from build123d import *

# Parameters (mm, degrees)
SKETCH1_W           = 165
SKETCH1_H           = 50.84
BOSS_EXTRUDE1_DEPTH = 10
SKETCH2_W           = 90
SKETCH2_H           = 10
BOSS_EXTRUDE2_DEPTH = 110
SKETCH3_R           = 4
CUT_EXTRUDE1_DEPTH  = 30
SKETCH4_W           = 90
SKETCH4_H           = 110
CUT_EXTRUDE2_DEPTH  = 0.5


with BuildPart() as part:
    # Sketch1 → Boss-Extrude1 (new body)
    with BuildSketch(Plane(origin=(0, 0, 0), x_dir=(1, 0, 0), z_dir=(0, 1, 0))):
        with Locations((82.5, 25.42)):
            Rectangle(SKETCH1_W, SKETCH1_H)
    extrude(amount=BOSS_EXTRUDE1_DEPTH)

    # Sketch2 → Boss-Extrude2 (add)
    with BuildSketch(Plane(origin=(0, 10, 0), x_dir=(1, 0, 0), z_dir=(0, 1, 0))):
        with Locations((80, 45.84)):
            Rectangle(SKETCH2_W, SKETCH2_H)
        with Locations((80, 5)):
            Rectangle(SKETCH2_W, SKETCH2_H)
    extrude(amount=BOSS_EXTRUDE2_DEPTH)

    # Sketch3 → Cut-Extrude1 (cut)
    with BuildSketch(Plane(origin=(0, 10, 0), x_dir=(1, 0, 0), z_dir=(0, 1, 0))):
        with Locations((30, 36.92)):
            Circle(SKETCH3_R)
        with Locations((155, 36.92)):
            Circle(SKETCH3_R)
    cut_extrude1 = extrude(amount=-CUT_EXTRUDE1_DEPTH, mode=Mode.SUBTRACT)

    # Mirror1: Cut-Extrude1 across plane
    add(cut_extrude1.mirror(Plane(origin=(0, 0, -25.42), x_dir=(1, 0, 0), z_dir=(0, 0, -1))), mode=Mode.SUBTRACT)

    # Sketch4 → Cut-Extrude2 (cut)
    with BuildSketch(Plane(origin=(0, 0, -10), x_dir=(-1, 0, 0), z_dir=(0, 0, -1))):
        with Locations((-80, 65)):
            Rectangle(SKETCH4_W, SKETCH4_H)
    cut_extrude2 = extrude(amount=-CUT_EXTRUDE2_DEPTH, mode=Mode.SUBTRACT)

    # Mirror2: Cut-Extrude2 across plane
    add(cut_extrude2.mirror(Plane(origin=(0, 0, -25.42), x_dir=(1, 0, 0), z_dir=(0, 0, -1))), mode=Mode.SUBTRACT)


solid = part.part
CAD build for the part. Positions are in the model's coordinates, mm. A direction names the side the tool comes from. Give positions to 0.01 mm unless a question says otherwise; leave off trailing zeros. Write each loop counter-clockwise with the first axis right and the second up, starting at its lowest first coordinate (ties: lowest second). Pieces come first, ordered by that corner, then holes. Notation, with made-up numbers: (56.5, 0) -> (78.5, 0) arc R17 cw to (78.5, 25) -> close; hole circle Ø4 at (-15, -7.5). An arc over 180 degrees is marked (long way). Return JSON: item names as keys, results as strings.
Item 1: Tool access for faces 4 (the flat face through (125, 64, -5)), 5 (the cylindrical face through (158.7, 5.1, -35.4)), 6 (the flat face through (81, 66, -41.34)), 7 (the flat face through (81, 0, -26)), 8 (the flat face through (35, 64, -46)): list every direction of +Z, -Z, +X, -X, +Y, -Y with a clear straight run to the whole face (end or side of a thin tool).
Answer below:
{"face 4": "+Z, -Z, +X, +Y", "face 5": "+Y, -Y", "face 6": "+X, -X, +Y", "face 7": "+Z, -Z, +X, -X, -Y", "face 8": "+Z, -Z, -X, +Y"}
Item 2: Two-plate mould, pull along X, no slides. Class faces 1 (the flat face through (165, 5, -25)), 2 (the flat face through (81, 10, -26)), 3 (the cylindrical face through (158.815, 5.07, -12.719)): +X half, -X half, draft (parallel to the pull), parting line (faces both ways), or undercut.
Answer below:
{"face 1": "+X half", "face 2": "draft", "face 3": "undercut"}
Item 3: Drop flat-ended pins along their axis: pin 1 (5 mm diameter, centred on y = 63.5, z = -46, fed in from +X); pin 2 (10.5 mm diameter, centred on x = 155, z = -13.92, fed in from +Y); pin 3 (10.5 mm diameter, centred on y = 61, z = -4.5, fed in from -X); pin 4 (10 mm diameter, centred on x = 26, y = 72, fed in from -Z). Give the stop position or say it passes through.
Answer below:
{"pin 1": "stops at x = 125", "pin 2": "stops at y = 10", "pin 3": "stops at x = 35", "pin 4": "passes through"}
Item 4: Band-saw the part on D-D (z = -13.92). List the corners of the cut face in (x, y).
Answer below:
{"outline": "(0, 0) -> (26, 0) -> (26, 10) -> (0, 10) -> close; (34, 0) -> (151, 0) -> (151, 10) -> (34, 10) -> close; (159, 0) -> (165, 0) -> (165, 10) -> (159, 10) -> close"}
Item 5: Band-saw the part on B-B (x = 30). List the corners of the cut face in (y, z), then the cut area to 3 significant figures.
Answer below:
{"outline": "(0, -50.84) -> (10, -50.84) -> (10, -40.92) -> (0, -40.92) -> close; (0, -32.92) -> (10, -32.92) -> (10, -17.92) -> (0, -17.92) -> close; (0, -9.92) -> (10, -9.92) -> (10, 0) -> (0, 0) -> close", "area": "348 mm2"}
Item 6: Drill centre lines: probe 1 along Z at (x, y) = (30, 5.25); probe 2 along X at (y, z) = (2.75, -36.92); probe 3 along X at (y, z) = (4, -36). Where is each one in solid material? Low to high.
Answer below:
{"probe 1": "z = -50.84 to -40.92, -32.92 to -17.92, -9.92 to 0", "probe 2": "x = 0 to 26, 34 to 151, 159 to 165", "probe 3": "x = 0 to 26.11, 33.89 to 151.11, 158.89 to 165"}
Item 7: Band-saw the part on C-C (z = -47.5). List the corners of the cut face in (x, y).
Answer below:
{"outline": "(0, 0) -> (165, 0) -> (165, 10) -> (125, 10) -> (125, 120) -> (35, 120) -> (35, 10) -> (0, 10) -> close"}
Item 8: Band-saw the part on A-A (y = 39). List the corners of the cut face in (x, z), then the cut area to 3 significant figures.
Answer below:
{"outline": "(35, -50.84) -> (125, -50.84) -> (125, -41.34) -> (35, -41.34) -> close; (35, -9.5) -> (125, -9.5) -> (125, 0) -> (35, 0) -> close", "area": "1,710 mm2"}
